Build history of the part. All positions in model axes, mm. Face numbers are marked on the shaded views. A direction names the side the tool comes from. Round coordinates to 2 decimals unless told otherwise and drop trailing zeros. Loops run counter-clockwise (first coordinate to the right, second up) from the corner with the lowest first, then second, coordinate; pieces in that order, holes last. Notation, with made-up numbers: (-2, 63) - (15, 63) arc R25 ccw to (15, 75) - close; hole circle Ø1 at (-33.5, 57). An arc over 180 degrees is marked (long way). Use one line per item in the form item = value. Start each with the question number.
Q1. Drill centre lines: line 1 (Z direction, x = 47, y = 40); line 2 (Z direction, x = 47.5, y = 39); line 3 (X direction, y = 4, z = 15). Where is each one in solid material? Low to high.
Q2. 3-axis set-ups, long thin cutter, end or side, ignore diameter. For the marked faces 1 and 2: which of +Z, -Z, +X, -X, +Y, -Y reach the whole face in a straight line?
Q3. Saw through at D-D (z = 21.5). Give the cut face in (x, y), then the cut area to 3 significant figures.
Q4. Saw through at A-A (z = -15). Give the cut face in (x, y), then the cut area to 3 significant figures.
Q5. Saw through at B-B (x = 10). Give the cut face in (y, z).
Q6. Mould opens along Y. For the marked faces 3, 4, 5 and 6 say: released by +Y, released by -Y, zero draft, split by the parting line, or undercut.
Q7. Saw through at C-C (y = 40). Give the cut face in (x, z).
Q8. Pin check, flat tips, straight feed: pin 1 (1.5 mm diameter, centred on x = 38, y = 27.5, fed in from -Z); pin 2 (5.5 mm diameter, centred on x = 31.5, z = -5.5, fed in from +Y); pin 3 (8.5 mm diameter, centred on y = 19, z = -2, fed in from -X); pin 4 (4 mm diameter, centred on x = 5, z = -17.5, fed in from +Y). Stop position of each tip, or through.
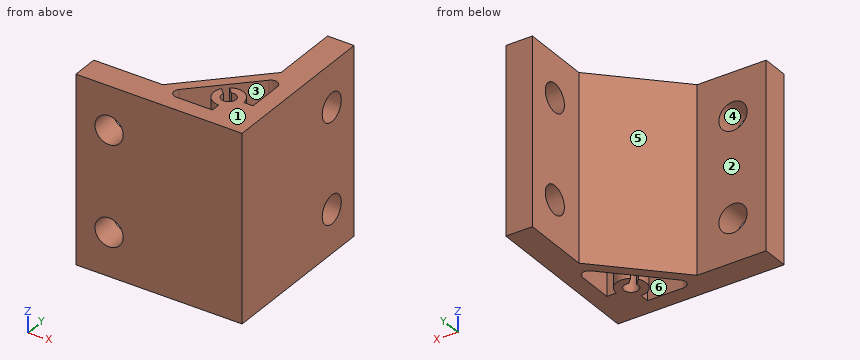
```python
from build123d import *

# Parameters (mm, degrees)
EXTRUDE_1_DEPTH     = 28
SKETCH_3_R          = 4.25
CUT_EXTRUDE_1_DEPTH = 56


with BuildPart() as part:
    # 草图1 → 凸台-拉伸1 (new, symmetric)
    with BuildSketch(Plane.XY):
        Polygon((0, 0), (50, 0), (50, 50), (42, 50), (42, 29.242640687), (20.757359313, 8), (0, 8), align=None)
        with BuildLine():
            Line((37.061279898, 14.352933665), (35.340960992, 16.07325257))
            ThreePointArc((35.340960992, 16.07325257), (39.856939547, 16.192314452), (42.15, 12.3))
            Line((42.15, 12.3), (45, 12.3))
            Line((45, 12.3), (45, 23.171572875))
            ThreePointArc((45, 23.171572875), (43.765366865, 25.01933194), (41.585786438, 24.585786438))
            Line((41.585786438, 24.585786438), (25.414213562, 8.414213562))
            ThreePointArc((25.414213562, 8.414213562), (24.98066806, 6.234633135), (26.828427125, 5))
            Line((26.828427125, 5), (37.7, 5))
            Line((37.7, 5), (37.7, 7.85))
            ThreePointArc((37.7, 7.85), (33.807685548, 10.143060453), (33.92674743, 14.659039008))
            Line((33.92674743, 14.659039008), (35.647066335, 12.938720102))
            ThreePointArc((35.647066335, 12.938720102), (39.22027958, 10.77972042), (37.061279898, 14.352933665))
        make_face(mode=Mode.SUBTRACT)
    extrude(amount=EXTRUDE_1_DEPTH, both=True)

    # 草图3 → 切除-拉伸1 (cut)
    with BuildSketch(Plane(origin=(0, 8, 0), x_dir=(1, 0, 0), z_dir=(0, 1, 0))):
        with Locations(Location((10, 15, 0), (0, 0, 270))):
            Circle(SKETCH_3_R)
        with Locations(Location((10, -15, 0), (0, 0, 270))):
            Circle(SKETCH_3_R)
    cut_extrude_1 = extrude(amount=-CUT_EXTRUDE_1_DEPTH, mode=Mode.SUBTRACT)

    # 镜向1: 切除-拉伸1 across plane
    add(cut_extrude_1.mirror(Plane(origin=(25, 25, 0), x_dir=(0, 0, 1), z_dir=(-0.7071067811865486, -0.7071067811865465, 0))), mode=Mode.SUBTRACT)


solid = part.part
```
Report:
q1.line_1 = -28 to -19.25, -10.75 to 10.75, 19.25 to 28
q1.line_2 = -28 to -19.13, -10.87 to 10.87, 19.13 to 28
q1.line_3 = 0 to 5.75, 14.25 to 50
q2.face_1 = +Z, +X, -X, +Y, -Y
q2.face_2 = +Z, -Z, -X, +Y
q3.outline = (0, 0) - (50, 0) - (50, 50) - (42, 50) - (42, 29.24) - (20.76, 8) - (0, 8) - close; hole (25.41, 8.41) arc R2 ccw to (26.83, 5) - (37.7, 5) - (37.7, 7.85) arc R4.45 cw to (33.93, 14.66) - (35.65, 12.94) arc R2.15 ccw (long way) to (37.06, 14.35) - (35.34, 16.07) arc R4.45 cw to (42.15, 12.3) - (45, 12.3) - (45, 23.17) arc R2 ccw to (41.59, 24.59) - close
q3.area = 788 mm²
q4.outline = (0, 0) - (5.75, 0) - (5.75, 8) - (0, 8) - close; (14.25, 0) - (50, 0) - (50, 35.75) - (42, 35.75) - (42, 29.24) - (20.76, 8) - (14.25, 8) - close; (42, 44.25) - (50, 44.25) - (50, 50) - (42, 50) - close; hole (25.41, 8.41) arc R2 ccw to (26.83, 5) - (37.7, 5) - (37.7, 7.85) arc R4.45 cw to (33.93, 14.66) - (35.65, 12.94) arc R2.15 ccw (long way) to (37.06, 14.35) - (35.34, 16.07) arc R4.45 cw to (42.15, 12.3) - (45, 12.3) - (45, 23.17) arc R2 ccw to (41.59, 24.59) - close
q4.area = 652 mm²
q5.outline = (0, -28) - (8, -28) - (8, -19.25) - (0, -19.25) - close; (0, -10.75) - (8, -10.75) - (8, 10.75) - (0, 10.75) - close; (0, 19.25) - (8, 19.25) - (8, 28) - (0, 28) - close
q6.face_3 = undercut
q6.face_4 = zero draft
q6.face_5 = released by +Y
q6.face_6 = undercut
q7.outline = (42, -28) - (50, -28) - (50, -19.25) - (42, -19.25) - close; (42, -10.75) - (50, -10.75) - (50, 10.75) - (42, 10.75) - close; (42, 19.25) - (50, 19.25) - (50, 28) - (42, 28) - close
q8.pin_1 = through
q8.pin_2 = 21.49
q8.pin_3 = 27.51
q8.pin_4 = 8
